from build123d import *

# Parameters (mm, degrees)
F6_DEPTH      = 114.3
F6_DEPTH_BACK = 114.3
F8_DEPTH      = 127.001
F8_DEPTH_BACK = 127.001
F9_W          = 279.4
F9_H          = 254
F10_DEPTH     = 2.54
F11_T         = -0.508


# Not quite as in the source:
# - a pattern or mirror of a feature is missing from the dataset's text; its kind, count and spacing are read off the source's solid


with BuildPart() as f6:
    # F5 (on Front) → F6 (new body, two sides)
    with BuildSketch(Plane.XZ) as f6_sk:
        Polygon((-76.2, 203.2), (-127, 0), (127, 0), (76.2, 203.2), (50.8, 203.2), (0, 11.3592253257), (-50.8, 203.2), align=None)
    extrude(amount=F6_DEPTH)
    extrude(f6_sk.sketch, amount=-F6_DEPTH_BACK)

    # F7 (on Right) → F8 (cut, two sides)
    with BuildSketch(Plane.YZ) as f8_sk:
        Polygon((-114.3, 203.2), (-114.3, 0), (-12.7, 203.2), align=None)
    f8 = extrude(amount=-F8_DEPTH, mode=Mode.SUBTRACT) + extrude(f8_sk.sketch, amount=F8_DEPTH_BACK, mode=Mode.SUBTRACT)

    # F8_copies: F8 across plane
    add(f8.mirror(Plane.ZX), mode=Mode.SUBTRACT)

    # F9 (on face) → F10 (join)
    with BuildSketch(Plane(origin=(0, 0, 0), x_dir=(1, 0, 0), z_dir=(0, 0, -1))):
        Rectangle(F9_W, F9_H)
    extrude(amount=F10_DEPTH)

    # F11
    f11_openings = [f6.faces().sort_by_distance(p)[0] for p in [
        (0, 0, -2.54),
        (63.5, 0, 203.2),
        (-63.5, 0, 203.2),
    ]]
    offset(amount=F11_T, openings=f11_openings, kind=Kind.INTERSECTION)


solid = f6.part
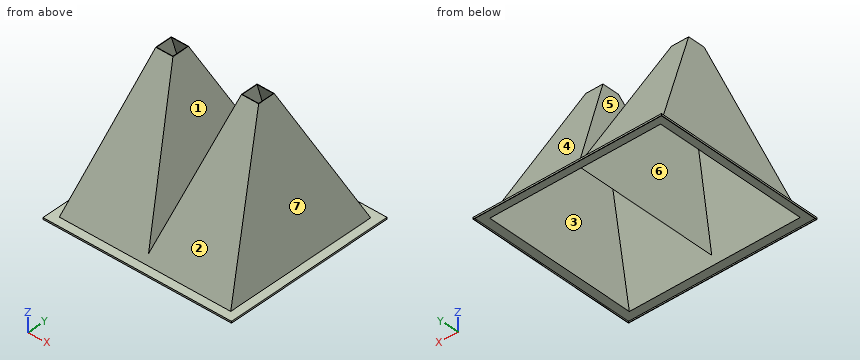
Can you work these out from the model? Positions are in its coordinate system, mm. Face numbers are marked on the shaded views. A direction names the side the tool comes from. Give positions to 0.01 mm unless a question says otherwise; leave off trailing zeros. Loops run counter-clockwise (first coordinate to the right, second up) from the corner with the lowest first, then second, coordinate; pieces in that order, holes last. Notation, with made-up numbers: (6, 70) -> (12, 70) arc R22 ccw to (12, 87) -> close; hole circle Ø10 at (66, 25). An arc over 180 degrees is marked (long way). Return JSON: item names as keys, results as strings.
Q1. I want a section at A-A, the plane z = 89.5. List the corners of the cut face in (x, y) for me (3 decimals).
Checks:
{"outline": "(-104.625, -69.55) -> (-20.692, -69.55) -> (-20.692, 69.55) -> (-104.625, 69.55) -> close; (20.692, -69.55) -> (104.625, -69.55) -> (104.625, 69.55) -> (20.692, 69.55) -> close; hole (-104.101, -68.982) -> (-21.217, -68.982) -> (-21.217, 68.982) -> (-104.101, 68.982) -> close; hole (21.217, -68.982) -> (104.101, -68.982) -> (104.101, 68.982) -> (21.217, 68.982) -> close"}
Q2. I need wall thicknesses on probe 1 along X at (y, z) = (43, 54); probe 2 along X at (y, z) = (54, 102.5) (3 decimals); probe 3 along Y at (x, z) = (47, 83). Which ranges of each line are inside material? Lowest first, please.
Checks:
{"probe 1": "x = -113.5 to -112.98, -11.82 to -11.29, 11.29 to 11.82, 112.98 to 113.5", "probe 2": "x = -101.375 to -100.851, -24.66 to -24.134, 24.134 to 24.66, 100.851 to 101.375", "probe 3": "y = -72.8 to -72.23, 72.23 to 72.8"}
Q3. We'd pull the mould along Y, two halves only. Please class the marked faces 1, 2, 3 and 4: released by +Y, released by -Y, zero draft, split by the parting line, or undercut.
Checks:
{"face 1": "zero draft", "face 2": "released by -Y", "face 3": "undercut", "face 4": "released by +Y"}
Q4. I want a section at B-B, the plane x = -71. List the corners of the cut face in (y, z) for me.
Checks:
{"outline": "(-127, -2.54) -> (-126.49, -2.54) -> (-126.49, -0.51) -> (-113.99, -0.51) -> (-12.13, 203.2) -> (-12.7, 203.2) -> (-114.3, 0) -> (-127, 0) -> close; (12.13, 203.2) -> (113.99, -0.51) -> (126.49, -0.51) -> (126.49, -2.54) -> (127, -2.54) -> (127, 0) -> (114.3, 0) -> (12.7, 203.2) -> close"}
Q5. I want a section at C-C, the plane z = 61. List the corners of the cut face in (x, y) for me, then the cut area to 3 significant figures.
Checks:
{"outline": "(-111.75, -83.8) -> (-13.15, -83.8) -> (-13.15, 83.8) -> (-111.75, 83.8) -> close; (13.15, -83.8) -> (111.75, -83.8) -> (111.75, 83.8) -> (13.15, 83.8) -> close; hole (-111.23, -83.23) -> (-13.67, -83.23) -> (-13.67, 83.23) -> (-111.23, 83.23) -> close; hole (13.67, -83.23) -> (111.23, -83.23) -> (111.23, 83.23) -> (13.67, 83.23) -> close", "area": "573 mm2"}
Q6. I want a section at D-D, the plane y = 63. List the corners of the cut face in (x, z) for me, then the cut area to 3 significant figures.
Checks:
{"outline": "(-139.7, -2.54) -> (-139.19, -2.54) -> (-139.19, -0.51) -> (-126.6, -0.51) -> (-101.11, 101.46) -> (-24.39, 101.46) -> (0, 9.37) -> (24.39, 101.46) -> (101.11, 101.46) -> (126.6, -0.51) -> (139.19, -0.51) -> (139.19, -2.54) -> (139.7, -2.54) -> (139.7, 0) -> (127, 0) -> (101.35, 102.6) -> (24.16, 102.6) -> (0, 11.36) -> (-24.16, 102.6) -> (-101.35, 102.6) -> (-127, 0) -> (-139.7, 0) -> close", "area": "393 mm2"}
Q7. On a 3-axis mill with a long thin cutter (end or side, diameter ignored), from which of +Z, -Z, +X, -X, +Y, -Y can I reach the whole of each face in a straight line? I mean the marked faces 5, 6 and 7. Say none if no direction works.
Checks:
{"face 5": "+Z, +Y, -Y", "face 6": "-Z", "face 7": "+Z, +X, +Y, -Y"}
Q8. For pin 1 Ø2 at (x, y) = (-74, 53.5) entering from -Z; pin 2 Ø8 at (x, y) = (26, 97.5) entering from -Z; pin 3 Ø2 at (x, z) = (65, 86.5) entering from -Y, each with a flat end and sliding along its axis, tell me the tip position at first contact or that it passes through.
Checks:
{"pin 1": "stops at z = 118.46", "pin 2": "stops at z = 24.46", "pin 3": "stops at y = -71.55"}
